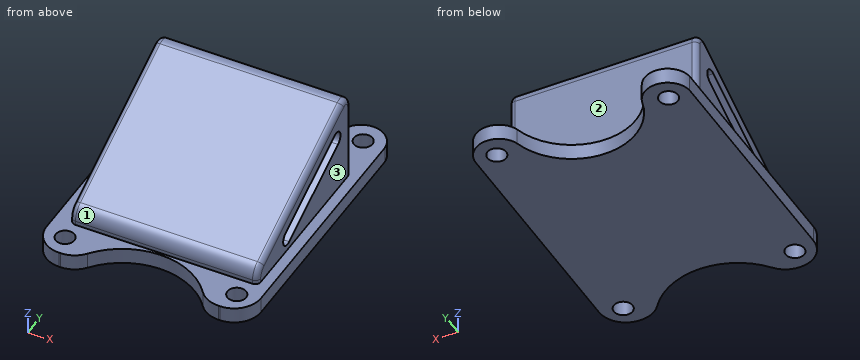
from build123d import *

# Parameters (mm, degrees)
F0_R     = 1.75
F1_DEPTH = 3
F3_DEPTH = 17.5
F4_R     = 1


with BuildPart() as f1:
    # F0 (on Top) → F1 (new body)
    with BuildSketch(Plane.XY):
        with BuildLine():
            ThreePointArc((-20.5195807586, -22.8886182085), (-19.0551146645, -26.4241521144), (-15.5195807586, -27.8886182085))
            Line((-15.5195807586, -27.8886182085), (-15.2333166803, -27.8886182085))
            ThreePointArc((-15.2333166803, -27.8886182085), (-13.0234939097, -27.3737807832), (-11.2687509252, -25.9352915373))
            ThreePointArc((-11.2687509252, -25.9352915373), (-0.5195807586, -20.639215731), (10.229589408, -25.9352915373))
            ThreePointArc((10.229589408, -25.9352915373), (11.9843323925, -27.3737807832), (14.1941551632, -27.8886182085))
            Line((14.1941551632, -27.8886182085), (14.4804192414, -27.8886182085))
            ThreePointArc((14.4804192414, -27.8886182085), (18.0159531473, -26.4241521144), (19.4804192414, -22.8886182085))
            Line((19.4804192414, -22.8886182085), (19.4804192414, 21.2272368371))
            ThreePointArc((19.4804192414, 21.2272368371), (15.7137853447, 25.1397413301), (11.1289973993, 22.2285659978))
            ThreePointArc((11.1289973993, 22.2285659978), (-0.5195807586, 13.1113817915), (-12.1681589164, 22.2285659978))
            ThreePointArc((-12.1681589164, 22.2285659978), (-16.7529468618, 25.1397413301), (-20.5195807586, 21.2272368371))
            Line((-20.5195807586, 21.2272368371), (-20.5195807586, -22.8886182085))
        make_face()
        with Locations((-16.5195807586, -23.8886182085)):
            Circle(F0_R, mode=Mode.SUBTRACT)
        with Locations((15.4804192414, -23.8886182085)):
            Circle(F0_R, mode=Mode.SUBTRACT)
        with Locations((-16.5195807586, 21.1113817915)):
            Circle(F0_R, mode=Mode.SUBTRACT)
        with Locations((15.4804192414, 21.1113817915)):
            Circle(F0_R, mode=Mode.SUBTRACT)
    extrude(amount=F1_DEPTH)

    # F2 (on Right) → F3 (join, symmetric)
    with BuildSketch(Plane.YZ):
        with BuildLine():
            Line((-20.2289633453, 3.7764561929), (-20.2289633453, 2.6880949736))
            Line((-20.2289633453, 2.6880949736), (12.7710366547, 2.6880949736))
            Line((12.7710366547, 2.6880949736), (12.7710366547, 17.9294266955))
            ThreePointArc((12.7710366547, 17.9294266955), (11.845807029, 19.6161005355), (9.9261680122, 19.7422137699))
            Line((9.9261680122, 19.7422137699), (-18.4962663091, 6.4956368044))
            ThreePointArc((-18.4962663091, 6.4956368044), (-19.7589741053, 5.3886117543), (-20.2289633453, 3.7764561929))
        make_face()
        with BuildLine():
            Line((-10.3537236473, 6.9807345733), (7.0411683064, 15.0878084597))
            ThreePointArc((7.0411683064, 15.0878084597), (9.0344100941, 14.3618696358), (8.3084712702, 12.3686278481))
            Line((8.3084712702, 12.3686278481), (-9.0864206835, 4.2615539618))
            ThreePointArc((-9.0864206835, 4.2615539618), (-11.0796624712, 4.9874927857), (-10.3537236473, 6.9807345733))
        make_face(mode=Mode.SUBTRACT)
    extrude(amount=F3_DEPTH, both=True)

    # F4
    f4_edges = [f1.edges().sort_by_distance(p)[0] for p in [
        (17.5, -4.285049, 13.118925),
        (-17.5, -4.285049, 13.118925),
    ]]
    fillet(f4_edges, radius=F4_R)


solid = f1.part
Model file for the job. Use its own axes, mm. Face numbers are marked on the shaded views. A direction names the side the tool comes from. Coordinates: 2 decimals unless noted, no trailing zeros. Order: outer loops, then holes, each group sorted by start corner. A loop starts at its lowest first (then second) coordinate and runs counter-clockwise, first axis right, second up. Notation, with made-up numbers: (86, -18.5) -> (131, -18.5) arc R5 cw to (131, -12.5) -> close; hole circle Ø8 at (-25, 51). An arc over 180 degrees is marked (long way). Return JSON: item names as keys, results as strings. Group by question number.
Item 1: Tool access for the marked faces 1, 2 and 3: list every direction of +Z, -Z, +X, -X, +Y, -Y with a clear straight run to the whole face (end or side of a thin tool).
Item 2: Flat gauge pins, fed straight in: P1, Ø4, axis at y = 5, z = 13.5, coming from the +X side; P2, Ø4.5, axis at x = 15.48, y = -23.89, coming from the +Z side; P3, Ø0.9, axis at x = 2, z = 3, coming from the -Y side. Where does each tip first touch, or does it go through?
Item 3: Saw through at B-B on x = -2.5. Write the cut outline in (y, z).
Item 4: Wall check: line 1 along X through (y, z) = (21.5, 2.25); line 2 along Z through (x, y) = (-11, 16); line 3 along X through (y, z) = (3, 7). Give the ranges that are in metal, low to high. Write a range as [from, to].
Item 5: Saw through at A-A on y = 15. Write the cut outline in (x, z), then the cut area to 3 significant figures.
Values found:
{
 "1": {"face 1": "+Z, +X, -X, -Y", "face 2": "+Z, +X, -X, +Y", "face 3": "+Z, +X, +Y, -Y"},
 "2": {"P1": "stops at x = 17.5", "P2": "stops at z = 3", "P3": "stops at y = -20.97"},
 "3": {"outline": "(-20.78, 0) -> (13.28, 0) -> (13.28, 3) -> (12.77, 3) -> (12.77, 17.93) arc R2 ccw to (9.93, 19.74) -> (-18.5, 6.5) arc R3 ccw to (-20.23, 3.78) -> (-20.23, 3) -> (-20.78, 3) -> close; hole (-10.35, 6.98) arc R1.5 ccw to (-9.09, 4.26) -> (8.31, 12.37) arc R1.5 ccw to (7.04, 15.09) -> close"},
 "4": {"line 1": "x = [-20.49, -18.23], [-14.81, -11.96], [10.92, 13.77], [17.19, 19.45]", "line 2": "z = [0, 3]", "line 3": "x = [-17.5, 17.5]"},
 "5": {"outline": "(-20.52, 0) -> (-6.98, 0) -> (-6.98, 3) -> (-20.52, 3) -> close; (5.94, 0) -> (19.48, 0) -> (19.48, 3) -> (5.94, 3) -> close", "area": "81.2 mm2"}
}
